from build123d import *

# Parameters (mm, degrees)
ESQUISSE3_R                  = 3.5
BOSS_EXTRU_1_DEPTH           = 25.65
ENL_V_MAT_EXTRU_2_DEPTH      = 58.051928101
ENL_V_MAT_EXTRU_2_DEPTH_BACK = 58.051928101
ESQUISSE5_W                  = 30
ESQUISSE5_H                  = 43.3
ENL_V_MAT_EXTRU_6_DEPTH      = 73.309681233
ESQUISSE20_W                 = 7
ESQUISSE20_H                 = 11.521668881
ENL_V_MAT_EXTRU_12_DEPTH     = 70.661251783
ESQUISSE22_R                 = 1
ENL_V_MAT_EXTRU_14_DEPTH     = 70.254348527
CONG_2_R                     = 5
ESQUISSE23_W                 = 24
ESQUISSE23_H                 = 36
ENL_V_MAT_EXTRU_15_DEPTH     = 15
CONG_3_R                     = 2


with BuildPart() as part:
    # Esquisse3 → Boss.-Extru.1 (new, symmetric)
    with BuildSketch(Plane(origin=(0, 0, 0), x_dir=(1, 0, 0), z_dir=(0, 1, 0))):
        with BuildLine():
            Line((-14, 0), (-14, -35))
            ThreePointArc((-14, -35), (0, -49), (14, -35))
            Line((14, -35), (14, 0))
            Line((14, 0), (-14, 0))
        make_face()
        with Locations(Location((0, -35, 0), (0, 0, 270))):
            Circle(ESQUISSE3_R, mode=Mode.SUBTRACT)
    extrude(amount=BOSS_EXTRU_1_DEPTH, both=True)

    # Esquisse5 → Enlèv. mat.-Extru.2 (cut, two sides: drawn at the far end of the back side and taken through both)
    with BuildSketch(Plane(origin=(0, 0, 0), x_dir=(0, 0, -1), z_dir=(1, 0, 0)).offset(-ENL_V_MAT_EXTRU_2_DEPTH_BACK)):
        with Locations((-34, 0)):
            Rectangle(ESQUISSE5_W, ESQUISSE5_H)
    extrude(amount=ENL_V_MAT_EXTRU_2_DEPTH + ENL_V_MAT_EXTRU_2_DEPTH_BACK, mode=Mode.SUBTRACT)

    # Esquisse11 → Enlèv. mat.-Extru.6 (cut, through all)
    with BuildSketch(Plane.XZ.offset(25.65)):
        with BuildLine():
            Line((14, 21.20346537), (14, 35))
            ThreePointArc((14, 35), (0, 49), (-14, 35))
            Line((-14, 35), (-14, 21.20346537))
            ThreePointArc((-14, 21.20346537), (-13.370879839, 23.757781245), (-11.627443785, 25.727743806))
            ThreePointArc((-11.627443785, 25.727743806), (-9.546893091, 28.483748084), (-9.519282304, 31.936788544))
            ThreePointArc((-9.519282304, 31.936788544), (0, 45), (9.519282304, 31.936788544))
            ThreePointArc((9.519282304, 31.936788544), (9.893665279, 28.601487898), (11.627443785, 25.727743806))
            ThreePointArc((11.627443785, 25.727743806), (13.370879839, 23.757781245), (14, 21.20346537))
        make_face()
    extrude(amount=-ENL_V_MAT_EXTRU_6_DEPTH, mode=Mode.SUBTRACT)

    # Esquisse20 → Enlèv. mat.-Extru.12 (cut, through all)
    with BuildSketch(Plane.XZ.offset(25.65)):
        with Locations((0, 40.760834441)):
            Rectangle(ESQUISSE20_W, ESQUISSE20_H)
    extrude(amount=-ENL_V_MAT_EXTRU_12_DEPTH, mode=Mode.SUBTRACT)

    # Esquisse22 → Enlèv. mat.-Extru.14 (cut, through all)
    with BuildSketch(Plane.XZ.offset(25.65)):
        with Locations(Location((0, 27.5, 0), (0, 0, 270))):
            Circle(ESQUISSE22_R)
        with Locations(Location((-7.5, 35, 0), (0, 0, 270))):
            Circle(ESQUISSE22_R)
        with Locations((0, 42.5)):
            Circle(ESQUISSE22_R)
        with Locations(Location((7.5, 35, 0), (0, 0, 270))):
            Circle(ESQUISSE22_R)
    extrude(amount=-ENL_V_MAT_EXTRU_14_DEPTH, mode=Mode.SUBTRACT)

    # Congé2
    cong_2_edges = [part.edges().sort_by_distance(p)[0] for p in [
        (0, -21.65, 19),
        (0, 21.65, 19),
    ]]
    fillet(cong_2_edges, radius=CONG_2_R)

    # Esquisse23 → Enlèv. mat.-Extru.15 (cut)
    with BuildSketch(Plane(origin=(0, 0, 0), x_dir=(-1, 0, 0), z_dir=(0, 0, -1))):
        Rectangle(ESQUISSE23_W, ESQUISSE23_H)
    extrude(amount=-ENL_V_MAT_EXTRU_15_DEPTH, mode=Mode.SUBTRACT)

    # Congé3
    cong_3_edges = [part.edges().sort_by_distance(p)[0] for p in [
        (-12, 0, 15),
        (-12, 18, 7.5),
        (0, -18, 15),
        (-12, -18, 7.5),
        (12, 0, 15),
        (12, -18, 7.5),
        (0, 18, 15),
        (12, 18, 7.5),
    ]]
    fillet(cong_3_edges, radius=CONG_3_R)


solid = part.part
Can you work these out from the model? Positions are in its coordinate system, mm. A direction names the side the tool comes from. Round coordinates to 2 decimals unless told otherwise and drop trailing zeros. Write each loop counter-clockwise with the first axis right and the second up, starting at its lowest first coordinate (ties: lowest second). Pieces come first, ordered by that corner, then holes. Notation, with made-up numbers: M -20.5,38.25 L 30.5,38.25 A8 cw 30.5,52.25 Z; hole C 61,44 d3. An arc over 180 degrees is marked long. Use CSV: the item, a comma, the result in double quotes.
(1) Imagine slicing it at D-D (x = -7.5). Write out the boundary of the cut face in (y, z), plus the area to 3 significant figures.
Check values:
outline,"M -25.65,0 L -18,0 L -18,13 A2 cw -16,15 L 16,15 A2 cw 18,13 L 18,0 L 25.65,0 L 25.65,34 L 21.65,34 L 21.65,24 A5 cw 16.65,19 L -16.65,19 A5 cw -21.65,24 L -21.65,34 L -25.65,34 Z; M -25.65,36 L -21.65,36 L -21.65,41.61 L -25.65,41.61 Z; M 21.65,36 L 25.65,36 L 25.65,41.61 L 21.65,41.61 Z"
area,"612 mm^2"
(2) Imagine slicing it at C-C (y = 8). Write out the boundary of the cut face in (x, z).
Check values:
outline,"M -14,0 L -12,0 L -12,13 A2 cw -10,15 L 10,15 A2 cw 12,13 L 12,0 L 14,0 L 14,19 L -14,19 Z"
(3) I'm going to push flat-ended pins straight in: pin 1 (5 mm diameter, centred on x = 3, y = 12.5, fed in from +Z); pin 2 (3 mm diameter, centred on y = 24, z = 38, fed in from -X); pin 3 (2.5 mm diameter, centred on x = -7.5, z = 35, fed in from +Y); pin 4 (2 mm diameter, centred on y = -24, z = 38, fed in from +X). Where does each tip first touch, or does it pass through?
Check values:
pin 1,"z = 19"
pin 2,"x = -9.89"
pin 3,"y = 25.65"
pin 4,"x = 9.8"
(4) I need wall thicknesses on line 1 along Y through (x, z) = (2.25, 4); line 2 along Y through (x, z) = (-4.5, 41); line 3 along X through (y, z) = (-4, 7). Which ranges of each line are inside material? Lowest first, please.
Check values:
line 1,"-25.65 to -18, 18 to 25.65"
line 2,"-25.65 to -21.65, 21.65 to 25.65"
line 3,"-14 to -12, 12 to 14"
(5) We'd pull the mould along X, two halves only. Please class faces 5 (the flat face through (-14, 0, 10)), 6 (the flat face through (13, 0, 0)), 7 (the cylindrical face through (-11.43, 0.22, 14.4)): +X half, -X half, draft (parallel to the pull), parting line (faces both ways), or undercut.
Check values:
face 5,"-X half"
face 6,"draft"
face 7,"undercut"
(6) Imagine slicing it at A-A (z = 22.5). Write out the boundary of the cut face in (x, y) (3 decimals).
Check values:
outline,"M -13.845,-25.65 L 13.845,-25.65 L 13.845,-21.42 L -13.845,-21.42 Z; M -13.845,21.42 L 13.845,21.42 L 13.845,25.65 L -13.845,25.65 Z"
(7) On a 3-axis mill with a long thin cutter (end or side, diameter ignored), from which of +Z, -Z, +X, -X, +Y, -Y can I reach the whole of each face in a straight line? I mean faces 1 (the cylindrical face through (0.2, -20.15, 20.43)), 2 (the cylindrical face through (8.953, -23.678, 39.454)), 3 (the cylindrical face through (11.43, 0.22, 14.4)), 4 (the flat face through (3.5, -24, 40)). Say none if no direction works.
Check values:
face 1,"+Z, +X, -X"
face 2,"+X, +Y, -Y"
face 3,"-Z"
face 4,"+Z, +Y, -Y"
(8) Imagine slicing it at B-B (z = 10.5). Write out the boundary of the cut face in (x, y).
Check values:
outline,"M -14,-25.65 L 14,-25.65 L 14,25.65 L -14,25.65 Z; hole M -12,-16 A2 ccw -10,-18 L 10,-18 A2 ccw 12,-16 L 12,16 A2 ccw 10,18 L -10,18 A2 ccw -12,16 Z"
